from build123d import *

# Parameters (mm, degrees)
CEOWNIK_C_100_X_10_1_DEPTH = 1750
OTW_R_13_2_13_2_1_D        = 13.2
OTW_R_13_2_13_2_1_DEPTH    = 51.034319914
OTW_R_13_2_13_2_1_TIP      = 3.965680086
OTW_R_9_2_9_2_1_D          = 9.2
OTW_R_9_2_9_2_1_DEPTH      = 52.236041152
OTW_R_9_2_9_2_1_TIP        = 2.763958848


with BuildPart() as part:
    # Sketch1 → Ceownik c 100 X 10(1) (new body)
    with BuildSketch(Plane(origin=(0, 0, 0), x_dir=(-1, 0, 0), z_dir=(0, 1, 0))):
        with BuildLine():
            Line((50, 100), (0, 100))
            Line((0, 100), (0, 0))
            Line((0, 0), (50, 0))
            Line((50, 0), (50, 1.629852671))
            ThreePointArc((50, 1.629852671), (48.844151715, 4.6409404), (45.970378085, 6.1052012))
            Line((45.970378085, 6.1052012), (13.063772294, 9.563824837))
            ThreePointArc((13.063772294, 9.563824837), (7.954841396, 12.166955149), (5.9, 17.52))
            Line((5.9, 17.52), (5.9, 82.48))
            ThreePointArc((5.9, 82.48), (7.954841396, 87.833044851), (13.063772294, 90.436175163))
            Line((13.063772294, 90.436175163), (45.970378085, 93.8947988))
            ThreePointArc((45.970378085, 93.8947988), (48.844151715, 95.3590596), (50, 98.370147329))
            Line((50, 98.370147329), (50, 100))
        make_face()
    extrude(amount=CEOWNIK_C_100_X_10_1_DEPTH)

    # Otwór Ø13.2 (13.2)1
    with Locations(Plane(origin=(0, 1608, 50), x_dir=(0, 0, 1), z_dir=(1, 0, 0))):
        with Locations((0, 0), (0, 315), (0, 1248)):
            Hole(OTW_R_13_2_13_2_1_D / 2, depth=OTW_R_13_2_13_2_1_DEPTH)
            with Locations((0, 0, -(OTW_R_13_2_13_2_1_DEPTH + OTW_R_13_2_13_2_1_TIP / 2))):  # 118° drill point
                Cone(0, OTW_R_13_2_13_2_1_D / 2, OTW_R_13_2_13_2_1_TIP, mode=Mode.SUBTRACT)

    # Otwór Ø9.2 (9.2)1
    with Locations(Plane(origin=(0, 1538, 50), x_dir=(0, 0, 1), z_dir=(1, 0, 0))):
        with Locations((0, 0), (0, -140), (0, 175), (0, 315), (0, 1108), (0, 1248)):
            Hole(OTW_R_9_2_9_2_1_D / 2, depth=OTW_R_9_2_9_2_1_DEPTH)
            with Locations((0, 0, -(OTW_R_9_2_9_2_1_DEPTH + OTW_R_9_2_9_2_1_TIP / 2))):  # 118° drill point
                Cone(0, OTW_R_9_2_9_2_1_D / 2, OTW_R_9_2_9_2_1_TIP, mode=Mode.SUBTRACT)


solid = part.part
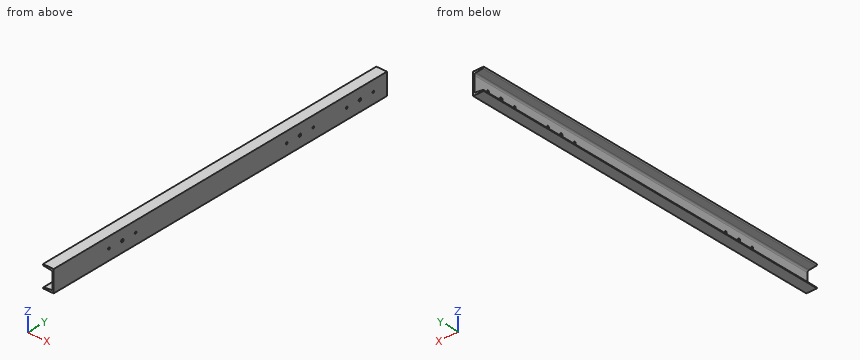
Geometry check sheet. Reference: the model listing, model coordinates, mm. Round coordinates to 2 decimals unless told otherwise and drop trailing zeros. Write each loop counter-clockwise with the first axis right and the second up, starting at its lowest first coordinate (ties: lowest second). Pieces come first, ordered by that corner, then holes. Notation, with made-up numbers: (-6, 88) -> (12, 88) arc R19 cw to (12, 123) -> close; hole circle Ø9 at (12, -33.75). An arc over 180 degrees is marked (long way). One line per item, written item: value. Start each with the question number.
(1) Cross-section at B-B, the plane x = -22. Record the cut outline in (y, z), and give its area (3 significant figures).
(2) Cross-section at A-A, the plane y = 1186.5. Record the cut outline in (x, z).
(3) Scan lines: line 1 (Z direction, x = -1, y = 290); line 2 (Z direction, x = -44, y = 537); line 3 (X direction, y = 1054, z = 63.5). Record each from-to range of solid material in increasing order. Write a range as [from, to].
(4) Go/stop test with a flat-tipped pin: pin 1 Ø10.5 at (y, z) = (290, 50) entering from -X. Record where the tip stops, or that it passes through.
Answer:
1. outline: (0, 0) -> (1750, 0) -> (1750, 8.62) -> (0, 8.62) -> close; (0, 91.38) -> (1750, 91.38) -> (1750, 100) -> (0, 100) -> close
1. area: 30,200 mm²
2. outline: (-50, 0) -> (0, 0) -> (0, 100) -> (-50, 100) -> (-50, 98.37) arc R4.5 ccw to (-45.97, 93.89) -> (-13.06, 90.44) arc R8 cw to (-5.9, 82.48) -> (-5.9, 17.52) arc R8 cw to (-13.06, 9.56) -> (-45.97, 6.11) arc R4.5 ccw to (-50, 1.63) -> close
3. line 1: [0, 45.4], [54.6, 100]
3. line 2: [0, 6.31], [93.69, 100]
3. line 3: [-5.9, 0]
4. pin 1: x = -5.9
